from build123d import *

# Parameters (mm, degrees)
F0_W     = 35.243742
F0_H     = 38.081205
F1_DEPTH = 25
F3_DEPTH = 10


with BuildPart() as f1:
    # F0 (on Top) → F1 (new body)
    with BuildSketch(Plane.XY):
        with Locations((-115.13764, -43.502171)):
            Rectangle(F0_W, F0_H)
    extrude(amount=F1_DEPTH)

    # F2 (on face) → F3 (cut)
    with BuildSketch(Plane.XZ.offset(62.542774)):
        Polygon((-115.13764, 25), (-97.515769, 12.5), (-97.515769, 25), align=None)
    extrude(amount=-F3_DEPTH, mode=Mode.SUBTRACT)


solid = f1.part
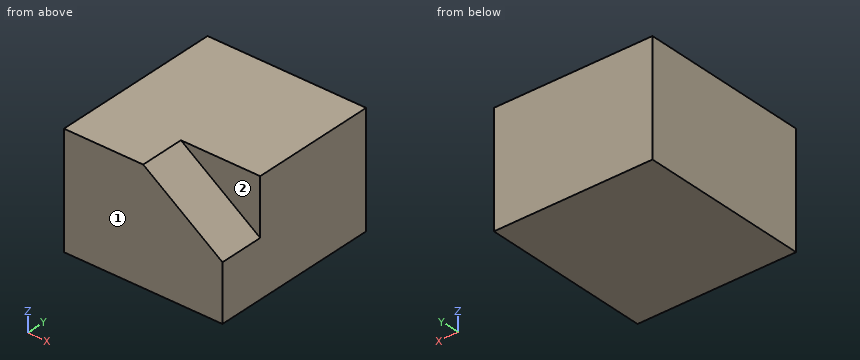
The model under review builds one solid part; all positions refer to its coordinate system, in mm. Face numbers are marked on the shaded views. A direction names the side the tool comes from. Round coordinates to 2 decimals unless told otherwise and drop trailing zeros. Write each loop counter-clockwise with the first axis right and the second up, starting at its lowest first coordinate (ties: lowest second). Pieces come first, ordered by that corner, then holes. Notation, with made-up numbers: M -14.75,-5 L 44.25,-5 A22 ccw 44.25,32 Z; hole C 68,9 d10. An arc over 180 degrees is marked long. Answer as CSV lines item,"result". Start each with the question number.
Q1. Consider section A-A, the plane z = 17.75. Give the boundary of the cut face in (x, y), then the cut area to 3 significant figures.
Q2. Consider section B-B, the plane x = -109. Give the boundary of the cut face in (y, z), then the cut area to 3 significant figures.
Q3. Tool access review of the marked faces 1 and 2: name each direction out of +Z, -Z, +X, -X, +Y, -Y from which nothing blocks a thin tool from reaching the whole face with its end or side.
Q4. Wall thickness on line 1 along X through (y, z) = (-58, 14.75); line 2 along X through (y, z) = (-59.5, 21.5); line 3 along Z through (x, y) = (-102, -55): over which ranges is each line inside the solid? List them lowest first.
Result set:
1,outline,"M -132.76,-62.54 L -104.92,-62.54 L -104.92,-52.54 L -97.52,-52.54 L -97.52,-24.46 L -132.76,-24.46 Z"
1,area,"1,270 mm²"
2,outline,"M -62.54,0 L -24.46,0 L -24.46,25 L -52.54,25 L -52.54,20.65 L -62.54,20.65 Z"
2,area,"908 mm²"
3,face 1,"+Z, -Z, +X, -X, -Y"
3,face 2,"+Z, +X, -Y"
4,line 1,"x = -132.76 to -100.69"
4,line 2,"x = -132.76 to -110.2"
4,line 3,"z = 0 to 15.68"
